```python
from build123d import *

# Parameters (mm, degrees)
F0_R     = 5
F0_R_2   = 14
F1_DEPTH = 12
F2_R     = 3
F3_DEPTH = 20
F5_DEPTH = 20


with BuildPart() as f1:
    # F0 (on Right) → F1 (new body)
    with BuildSketch(Plane.YZ):
        Polygon((-50, 43.5), (0, 0), (240, 0), (260, 43.5), (240, 87), (0, 87), align=None)
        with Locations((66.5, 43.5)):
            Circle(F0_R, mode=Mode.SUBTRACT)
        with Locations((126.5, 43.5)):
            Circle(F0_R_2, mode=Mode.SUBTRACT)
        with Locations((191.5, 43.5)):
            Circle(F0_R, mode=Mode.SUBTRACT)
    extrude(amount=F1_DEPTH)

    # F2 (on face) → F3 (cut)
    with BuildSketch(Plane.XY.offset(87)):
        with Locations((6, 13)):
            Circle(F2_R)
        with Locations((6, 43)):
            Circle(F2_R)
        with Locations((6, 73)):
            Circle(F2_R)
        with Locations((6, 103)):
            Circle(F2_R)
        with Locations((6, 133)):
            Circle(F2_R)
        with Locations((6, 163)):
            Circle(F2_R)
        with Locations((6, 193)):
            Circle(F2_R)
        with Locations((6, 223)):
            Circle(F2_R)
    extrude(amount=-F3_DEPTH, mode=Mode.SUBTRACT)

    # F4 (on face) → F5 (cut)
    with BuildSketch(Plane(origin=(0, 0, 0), x_dir=(1, 0, 0), z_dir=(0, 0, -1))):
        with BuildLine():
            ThreePointArc((6, -220), (3, -223), (6, -226))
            Line((6, -226), (6, -220))
        make_face()
        with BuildLine():
            ThreePointArc((6, -10), (3, -13), (6, -16))
            Line((6, -16), (6, -13))
            Line((6, -13), (6, -10))
        make_face()
        with BuildLine():
            Line((6, -13), (6, -16))
            ThreePointArc((6, -16), (8.12132, -15.12132), (9, -13))
            Line((9, -13), (6, -13))
        make_face()
        with BuildLine():
            ThreePointArc((6, -40), (3, -43), (6, -46))
            Line((6, -46), (6, -43))
            Line((6, -43), (6, -40))
        make_face()
        with BuildLine():
            Line((6, -43), (6, -46))
            ThreePointArc((6, -46), (8.12132, -45.12132), (9, -43))
            ThreePointArc((9, -43), (8.12132, -40.87868), (6, -40))
            Line((6, -40), (6, -43))
        make_face()
        with BuildLine():
            ThreePointArc((6, -70), (3, -73), (6, -76))
            Line((6, -76), (6, -70))
        make_face()
        with BuildLine():
            Line((6, -70), (6, -76))
            ThreePointArc((6, -76), (8.12132, -75.12132), (9, -73))
            ThreePointArc((9, -73), (8.12132, -70.87868), (6, -70))
        make_face()
        with BuildLine():
            ThreePointArc((6, -100), (3, -103), (6, -106))
            Line((6, -106), (6, -100))
        make_face()
        with BuildLine():
            Line((6, -100), (6, -106))
            ThreePointArc((6, -106), (8.12132, -105.12132), (9, -103))
            ThreePointArc((9, -103), (8.12132, -100.87868), (6, -100))
        make_face()
        with BuildLine():
            ThreePointArc((6, -130), (3, -133), (6, -136))
            Line((6, -136), (6, -130))
        make_face()
        with BuildLine():
            Line((6, -130), (6, -136))
            ThreePointArc((6, -136), (8.12132, -135.12132), (9, -133))
            ThreePointArc((9, -133), (8.12132, -130.87868), (6, -130))
        make_face()
        with BuildLine():
            ThreePointArc((6, -160), (3, -163), (6, -166))
            Line((6, -166), (6, -160))
        make_face()
        with BuildLine():
            Line((6, -160), (6, -166))
            ThreePointArc((6, -166), (8.12132, -165.12132), (9, -163))
            ThreePointArc((9, -163), (8.12132, -160.87868), (6, -160))
        make_face()
        with BuildLine():
            ThreePointArc((6, -190), (3, -193), (6, -196))
            Line((6, -196), (6, -190))
        make_face()
        with BuildLine():
            Line((6, -190), (6, -196))
            ThreePointArc((6, -196), (8.12132, -195.12132), (9, -193))
            ThreePointArc((9, -193), (8.12132, -190.87868), (6, -190))
        make_face()
        with BuildLine():
            Line((6, -220), (6, -226))
            ThreePointArc((6, -226), (8.12132, -225.12132), (9, -223))
            ThreePointArc((9, -223), (8.12132, -220.87868), (6, -220))
        make_face()
        with BuildLine():
            Line((6, -10), (6, -13))
            Line((6, -13), (9, -13))
            ThreePointArc((9, -13), (8.12132, -10.87868), (6, -10))
        make_face()
    extrude(amount=-F5_DEPTH, mode=Mode.SUBTRACT)


solid = f1.part
```
CAD build for the part. Positions are in the model's coordinates, mm. A direction names the side the tool comes from. Coordinates: 2 decimals unless noted, no trailing zeros. Write each loop counter-clockwise with the first axis right and the second up, starting at its lowest first coordinate (ties: lowest second). Pieces come first, ordered by that corner, then holes. Notation, with made-up numbers: (19, 63) -> (54, 63) arc R33 cw to (54, 98) -> close; hole circle Ø2 at (24.25, 28). An arc over 180 degrees is marked (long way). Use CSV: the item, a comma, the result in double quotes. Start each with the question number.
Item 1: Band-saw the part on A-A, the plane y = 66.5. Write the cut outline in (x, z), plus the area to 3 significant figures.
Item 2: Drop flat-ended pins along their axis: P1, Ø5, axis at x = 6, y = 133, coming from the +Z side; P2, Ø5, axis at x = 5, z = 61, coming from the +Y side; P3, Ø1, axis at x = 2.5, z = 50, coming from the +Y side; P4, Ø22.5, axis at y = 126.5, z = 43.5, coming from the +X side. Give the stop position or say it passes through.
Item 3: Tool access for faces 4 (the flat face through (6, 163, 20)), 5 (the flat face through (6, 133, 67)), 6 (the flat face through (5.916, -24.65, 65.554)): list every direction of +Z, -Z, +X, -X, +Y, -Y with a clear straight run to the whole face (end or side of a thin tool).
Item 4: Wall check: probe 1 along Z at (x, y) = (4, 191.5); probe 2 along X at (y, z) = (193, 74.75); probe 3 along X at (y, z) = (161.5, 12). Give the ranges that are in metal, low to high.
Item 5: Two-plate mould, pull along Y, no slides. Class faces 1 (the flat face through (6, 118, 0)), 2 (the cylindrical face through (6, 226, 77)), 3 (the flat face through (5.916, -25.35, 22.054)): +Y half, -Y half, draft (parallel to the pull), parting line (faces both ways), or undercut.
Item 6: Band-saw the part on B-B, the plane z = 77.5. Give the number of separate pieces and of enclosed holes in the cut face, plus the area to 3 significant figures.
Item 7: Band-saw the part on C-C, the plane y = 126.5. Write the cut outline in (x, z), plus the area to 3 significant figures.
Response values:
1,outline,"(0, 0) -> (12, 0) -> (12, 38.5) -> (0, 38.5) -> close; (0, 48.5) -> (12, 48.5) -> (12, 87) -> (0, 87) -> close"
1,area,"924 mm2"
2,P1,"stops at z = 67"
2,P2,"stops at y = 253.1"
2,P3,"stops at y = 257.24"
2,P4,"passes through"
3,face 4,"-Z"
3,face 5,"+Z"
3,face 6,"+Z, +X, -X, -Y"
4,probe 1,"z = 20 to 38.5, 48.5 to 67"
4,probe 2,"x = 0 to 3, 9 to 12"
4,probe 3,"x = 0 to 3.4, 8.6 to 12"
5,face 1,"draft"
5,face 2,"undercut"
5,face 3,"-Y half"
6,separate pieces,"1"
6,enclosed holes,"8"
6,area,"2,840 mm2"
7,outline,"(0, 0) -> (12, 0) -> (12, 29.5) -> (0, 29.5) -> close; (0, 57.5) -> (12, 57.5) -> (12, 87) -> (0, 87) -> close"
7,area,"708 mm2"
